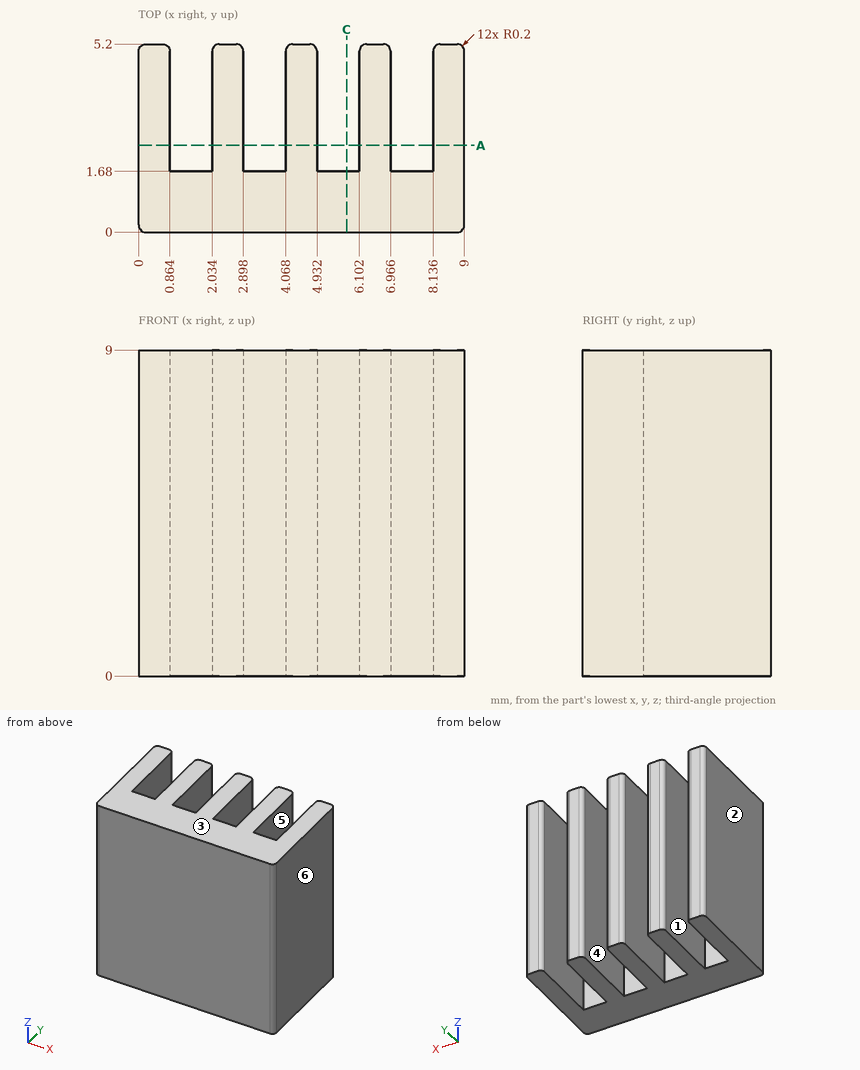
Geometry check sheet. Reference: drawing and pictorial views, mm from the part's lowest x, y, z. A direction names the side the tool comes from. Coordinates: 2 decimals unless noted, no trailing zeros. Order: outer loops, then holes, each group sorted by start corner. A loop starts at its lowest first (then second) coordinate and runs counter-clockwise, first axis right, second up.
1. Sectioned sample at A-A, the plane y = 2.4. Record the cut outline in (x, z).
Results found:
outline: (0, 0) - (0.86, 0) - (0.86, 9) - (0, 9) - close; (2.03, 0) - (2.9, 0) - (2.9, 9) - (2.03, 9) - close; (4.07, 0) - (4.93, 0) - (4.93, 9) - (4.07, 9) - close; (6.1, 0) - (6.97, 0) - (6.97, 9) - (6.1, 9) - close; (8.14, 0) - (9, 0) - (9, 9) - (8.14, 9) - close
2. Sectioned sample at C-C, the plane x = 5.75. Record the cut outline in (y, z), and give its area (3 significant figures).
Results found:
outline: (0, 0) - (1.68, 0) - (1.68, 9) - (0, 9) - close
area: 15.1 mm2
3. Scan lines: line 1 (X direction, y = 3.8, z = 5.5); line 2 (Y direction, x = 4, z = 8). Record each from-to range of solid material in increasing order.
Results found:
line 1: x = 0 to 0.86, 2.03 to 2.9, 4.07 to 4.93, 6.1 to 6.97, 8.14 to 9
line 2: y = 0 to 1.68
4. Set-up check for the marked faces 1 and 2: record each of +Z, -Z, +X, -X, +Y, -Y from which the full face is reachable in a straight line by a thin tool's end or side.
Results found:
face 1: +Z, -Z, +Y
face 2: +Z, -Z, -X, +Y, -Y
5. Release check for a two-part mould opening along X. For the marked faces 3, 4, 5 and 6 record: +X half, -X half, draft (parallel to the pull), parting line (faces both ways), or undercut.
Results found:
face 3: draft
face 4: undercut
face 5: undercut
face 6: +X half
